Read the model definition and answer for the solid it produces. Units are mm, in the model's axes. A direction names the side the tool comes from. Give positions to 0.01 mm unless a question says otherwise; leave off trailing zeros. Order: outer loops, then holes, each group sorted by start corner. A loop starts at its lowest first (then second) coordinate and runs counter-clockwise, first axis right, second up. Notation, with made-up numbers: (26.5, 20.25) -> (74.5, 20.25) arc R15 ccw to (74.5, 49.25) -> close; hole circle Ø3 at (-15.75, -15). An arc over 180 degrees is marked (long way). Answer as CSV lines item,"result". Start each with the question number.
1) For faces 1 (the face through (-272, 259, -456.307)), 2 (the face through (310, 0, 140)), determine the directions among +Z, -Z, +X, -X, +Y, -Y from which every point of the face is accessible in a straight line to the end or side of a thin tool.
2) Straight lines are drawn through the part: L1, parallel to Y at x = 262.5, z = 1; L2, parallel to X at y = 12, z = -367.5; L3, parallel to X at y = 242.5, z = 195. For each, find the intervals that lie inside material, in ascending order. Write a range as from..to.
3) The mould has two halves that part along Z. Classify faces 3 (the face through (125.78, 300.53, 365.29)), 4 (the face through (-757.281, 259, 124)), 5 (the face through (-272, 259, 720.485)): +Z half, -Z half, draft (parallel to the pull), parting line (faces both ways), or undercut.
4) Flat-ended cylindrical pins translate along their axes: pin 1 Ø1 at (y, z) = (424, 198.5) entering from +X; pin 2 Ø10 at (y, z) = (2, 591.5) entering from +X. Find the tip coordinate at first contact, or state that the pin passes through.
5) Find section D-D (x = 268.5). Determine the outline of the cut face in (y, z), and give its area (3 significant figures).
6) Find section C-C (z = -99). Determine the outline of the cut face in (x, y).
7) Find section B-B (x = 82). Determine the outline of the cut face in (y, z), and give its area (3 significant figures).
8) Find section A-A (y = 419). Determine the outline of the cut face in (x, z), and give its area (3 significant figures).
```python
from build123d import *

# Parameters (mm, degrees)
BOSS_EXTRUDE1_DEPTH = 609.6
SKETCH2_W           = 1270
SKETCH2_H           = 1176.792419191
BOSS_EXTRUDE2_DEPTH = 101.6


with BuildPart() as part:
    # Sketch1 → Boss-Extrude1 (new body)
    with BuildSketch(Plane(origin=(0, 0, 0), x_dir=(1, 0, 0), z_dir=(0, 1, 0))):
        Polygon((0, 0), (157.119191341, 456.307264584), (-757.280808659, 456.307264584), (-757.280808659, -720.485154607), (248.082933696, -720.485154607), align=None)
    extrude(amount=BOSS_EXTRUDE1_DEPTH)

    # Sketch2 → Boss-Extrude2 (add)
    with BuildSketch(Plane.XZ):
        with Locations((-122.280808659, 132.088945011)):
            Rectangle(SKETCH2_W, SKETCH2_H)
    extrude(amount=BOSS_EXTRUDE2_DEPTH)


solid = part.part
```
Findings below:
1,face 1,"-Z, +X, -X, +Y, -Y"
1,face 2,"+X, +Y"
2,L1,"-101.6..0"
2,L2,"-757.28..126.54"
2,L3,"-757.28..67.14"
3,face 3,"undercut"
3,face 4,"draft"
3,face 5,"+Z half"
4,pin 1,"x = 68.52"
4,pin 2,"x = 512.72"
5,outline,"(-101.6, -456.31) -> (0, -456.31) -> (0, 720.49) -> (-101.6, 720.49) -> close"
5,area,"120,000 mm²"
6,outline,"(-757.28, -101.6) -> (512.72, -101.6) -> (512.72, 0) -> (34.09, 0) -> (34.09, 609.6) -> (-757.28, 609.6) -> close"
7,outline,"(-101.6, -456.31) -> (609.6, -456.31) -> (609.6, -238.15) -> (0, -238.15) -> (0, 238.15) -> (609.6, 238.15) -> (609.6, 720.49) -> (-101.6, 720.49) -> close"
7,area,"547,000 mm²"
8,outline,"(-757.28, -456.31) -> (157.12, -456.31) -> (0, 0) -> (248.08, 720.49) -> (-757.28, 720.49) -> close"
8,area,"1,020,000 mm²"
